from build123d import *

# Parameters (mm, degrees)
SKETCH_1_W          = 4
SKETCH_1_H          = 5
EXTRUDE_1_DEPTH     = 6
SKETCH_4_W          = 1.2
SKETCH_4_H          = 5
EXTRUDE_2_DEPTH     = 5
SKETCH_5_W          = 1.2
SKETCH_5_H          = 5
EXTRUDE_3_DEPTH     = 3.5
FILLET_1_R          = 1
SKETCH_6_R          = 1.5
CUT_EXTRUDE_1_DEPTH = 10.552486587
FILLET_2_R          = 0.5


with BuildPart() as part:
    # 草图1 → 凸台-拉伸1 (new body)
    with BuildSketch(Plane.XY):
        Rectangle(SKETCH_1_W, SKETCH_1_H)
    extrude(amount=EXTRUDE_1_DEPTH)

    # 草图4 → 凸台-拉伸2 (add)
    with BuildSketch(Plane(origin=(2, 0, 0), x_dir=(0, 0, -1), z_dir=(1, 0, 0))):
        with Locations((-5.4, 0)):
            Rectangle(SKETCH_4_W, SKETCH_4_H)
    extrude(amount=EXTRUDE_2_DEPTH)

    # 草图5 → 凸台-拉伸3 (add)
    with BuildSketch(Plane(origin=(0, 0, 4.8), x_dir=(-1, 0, 0), z_dir=(0, 0, -1))):
        with Locations((-6.4, 0)):
            Rectangle(SKETCH_5_W, SKETCH_5_H)
    extrude(amount=EXTRUDE_3_DEPTH)

    # 圆角1
    fillet_1_edges = [part.edges().sort_by_distance(p)[0] for p in [
        (7, 0, 6),
    ]]
    fillet(fillet_1_edges, radius=FILLET_1_R)

    # 草图6 → 切除-拉伸1 (cut, through all)
    with BuildSketch(Plane.XY.offset(6)):
        Circle(SKETCH_6_R)
    extrude(amount=-CUT_EXTRUDE_1_DEPTH, mode=Mode.SUBTRACT)

    # 圆角2
    fillet_2_edges = [part.edges().sort_by_distance(p)[0] for p in [
        (-2, 0, 6),
    ]]
    fillet(fillet_2_edges, radius=FILLET_2_R - 0.0001)  # a hair under: the kernel refuses the full size


solid = part.part
Geometry check sheet. Reference: the model listing, model coordinates, mm. A direction names the side the tool comes from. Coordinates: 2 decimals unless noted, no trailing zeros. Loops run counter-clockwise (first coordinate to the right, second up) from the corner with the lowest first, then second, coordinate; pieces in that order, holes last. Notation, with made-up numbers: (-3, 3.5) - (28, 3.5) arc R19 cw to (28, 19.5) - close; hole circle Ø11 at (9, 40). An arc over 180 degrees is marked (long way). Use one line per item in the form item = value. Start each with the question number.
Item 1: Gauge pin test, flat end, axial feed: pin 1 (3 mm diameter, centred on x = 4, y = -1, fed in from -Z). Record the tip position at first contact, or that the pin passes through.
Item 2: Section check D-D, the plane y = -2.1. Enter the section's corners in (x, z).
Item 3: Thickness scan on probe 1 along Y at (x, z) = (0, 3.3); probe 2 along X at (y, z) = (-2.05, 4.35); probe 3 along X at (y, z) = (0.5, 3.7). Record the ranges inside material, lowest first.
Item 4: Tool access check on faces 1 (the face through (6, 0, 1.3)), 2 (the face through (5.8, 0, 3)), 3 (the face through (7, 0, 3)). Record the directions out of +Z, -Z, +X, -X, +Y, -Y that give a thin tool (end or side, any length) a straight path to the whole face; none if there is none.
Item 5: Section check A-A, the plane z = 4.55. Enter the section's corners in (x, y).
Item 6: Section check C-C, the plane x = 0. Enter the section's corners in (y, z).
Computed:
q1.pin_1 = 4.8
q2.outline = (-2, 0) - (2, 0) - (2, 4.8) - (5.8, 4.8) - (5.8, 1.3) - (7, 1.3) - (7, 5) arc R1 ccw to (6, 6) - (-1.5, 6) arc R0.5 ccw to (-2, 5.5) - close
q3.probe_1 = -2.5 to -1.5, 1.5 to 2.5
q3.probe_2 = -2 to 2, 5.8 to 7
q3.probe_3 = -2 to -1.41, 1.41 to 2, 5.8 to 7
q4.face_1 = -Z, +X, +Y, -Y
q4.face_2 = -Z, +Y, -Y
q4.face_3 = +Z, -Z, +X, +Y, -Y
q5.outline = (-2, -2.5) - (2, -2.5) - (2, 2.5) - (-2, 2.5) - close; (5.8, -2.5) - (7, -2.5) - (7, 2.5) - (5.8, 2.5) - close; hole circle Ø3 at (0, 0)
q6.outline = (-2.5, 0) - (-1.5, 0) - (-1.5, 6) - (-2.5, 6) - close; (1.5, 0) - (2.5, 0) - (2.5, 6) - (1.5, 6) - close
